from build123d import *

# Parameters (mm, degrees)
F1_DEPTH  = 25.4
F2_W      = 152.4
F2_H      = 152.4
F3_DEPTH  = 152.4
F4_R      = 25.4
F5_DEPTH  = 152.401
F6_W      = 152.4
F6_H      = 38.1
F7_DEPTH  = 152.4
F8_R      = 12.7
F9_DEPTH  = 133.351
F11_DEPTH = 152.4


with BuildPart() as f1:
    # F0 (on Top) → F1 (new body)
    with BuildSketch(Plane.XY):
        Polygon((304.8, 152.4), (-304.8, 152.4), (-304.8, 0), (-304.8, -152.4), (304.8, -152.4), align=None)
    extrude(amount=-F1_DEPTH)

    # F2 (on face) → F3 (join)
    with BuildSketch(Plane.XY):
        with Locations((-228.6, 0)):
            Rectangle(F2_W, F2_H)
    extrude(amount=F3_DEPTH)

    # F4 (on face) → F5 (cut, through all)
    with BuildSketch(Plane.YZ.offset(-152.4)):
        with Locations((0, 114.3)):
            Circle(F4_R)
    extrude(amount=-F5_DEPTH, mode=Mode.SUBTRACT)

    # F6 (on face) → F7 (join)
    with BuildSketch(Plane.XY):
        with Locations((228.6, 38.1)):
            Rectangle(F6_W, F6_H)
    extrude(amount=F7_DEPTH)

    # F8 (on face) → F9 (cut, through all)
    with BuildSketch(Plane.XZ.offset(-19.05)):
        with Locations((228.6, 114.3)):
            Circle(F8_R)
    extrude(amount=-F9_DEPTH, mode=Mode.SUBTRACT)

    # F10 (on face) → F11 (join, through all)
    with BuildSketch(Plane.YZ.offset(-152.4)):
        with BuildLine():
            Line((-76.2, 152.4), (76.2, 152.4))
            ThreePointArc((76.2, 152.4), (0, 184.260238), (-76.2, 152.4))
        make_face()
    extrude(amount=-F11_DEPTH)


solid = f1.part
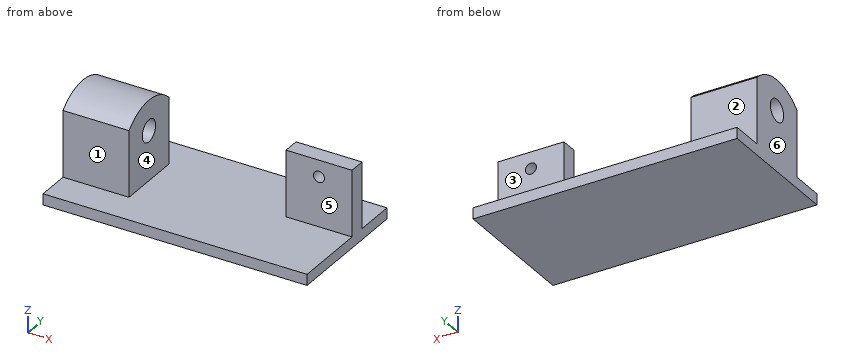
Input: part model. Units: mm. Frame: model coordinates. Face numbers are marked on the shaded views. A direction names the side the tool comes from. Coordinates: 2 decimals unless noted, no trailing zeros. Loops run counter-clockwise (first coordinate to the right, second up) from the corner with the lowest first, then second, coordinate; pieces in that order, holes last. Notation, with made-up numbers: (-23.5, 79.5) - (33.5, 79.5) arc R27 ccw to (33.5, 97.5) - close; hole circle Ø3 at (57, 66.5). An arc over 180 degrees is marked (long way). Answer in a Markdown table with one row per item. Add a question column.
Item 1: Mould query, pull axis X, two halves, no side actions, for the marked faces 4, 5 and 6. Classes: released by +X, released by -X, zero draft, split by the parting line, or undercut.
Item 2: Section query D-D on z = 50. Return the cut outline in (x, y).
Item 3: Line query: line 1 along X through (y, z) = (45, 114); line 2 along X through (y, z) = (35, 14); line 3 along Y through (x, z) = (-243, 114). Output: solid intervals per line, ascending. Write a range as [from, to].
Item 4: Access query for the marked faces 1, 2 and 3. Directions: +Z, -Z, +X, -X, +Y, -Y. A direction counts if a zero-diameter tool reaches every point of the face in a straight line with its end or side. Return the directions, or none.
Item 5: Section query A-A on x = 228.6. Return the cut outline in (y, z).
Item 6: Section query C-C on y = 0. Return the cut outline in (x, z), then the cut area to 3 significant figures.
Item 7: Section query B-B on z = 114.3. Return the cut outline in (x, y).
Item 8: Contact query for a flat-ended pin moving along its axis: P1, Ø8, axis at y = -30.5, z = 25.5, coming from the +X side. Output: stop coordinate, or through.
Recorded:
| question | item | result |
|---|---|---|
| 1 | face 4 | undercut |
| 1 | face 5 | zero draft |
| 1 | face 6 | released by -X |
| 2 | outline | (-304.8, -76.2) - (-152.4, -76.2) - (-152.4, 76.2) - (-304.8, 76.2) - close; (152.4, 19.05) - (304.8, 19.05) - (304.8, 57.15) - (152.4, 57.15) - close |
| 3 | line 1 | [-304.8, -152.4], [152.4, 215.9], [241.3, 304.8] |
| 3 | line 2 | [-304.8, -152.4], [152.4, 304.8] |
| 3 | line 3 | [-76.2, -25.4], [25.4, 76.2] |
| 4 | face 1 | +Z, +X, -X, -Y |
| 4 | face 2 | +Z, +X, -X, +Y |
| 4 | face 3 | +Z, +X, +Y |
| 5 | outline | (-152.4, -25.4) - (152.4, -25.4) - (152.4, 0) - (57.15, 0) - (57.15, 101.6) - (19.05, 101.6) - (19.05, 0) - (-152.4, 0) - close; (19.05, 127) - (57.15, 127) - (57.15, 152.4) - (19.05, 152.4) - close |
| 6 | outline | (-304.8, -25.4) - (304.8, -25.4) - (304.8, 0) - (-152.4, 0) - (-152.4, 88.9) - (-304.8, 88.9) - close; (-304.8, 139.7) - (-152.4, 139.7) - (-152.4, 184.26) - (-304.8, 184.26) - close |
| 6 | area | 35,800 mm^2 |
| 7 | outline | (-304.8, -76.2) - (-152.4, -76.2) - (-152.4, -25.4) - (-304.8, -25.4) - close; (-304.8, 25.4) - (-152.4, 25.4) - (-152.4, 76.2) - (-304.8, 76.2) - close; (152.4, 19.05) - (215.9, 19.05) - (215.9, 57.15) - (152.4, 57.15) - close; (241.3, 19.05) - (304.8, 19.05) - (304.8, 57.15) - (241.3, 57.15) - close |
| 8 | P1 | x = -152.4 |
